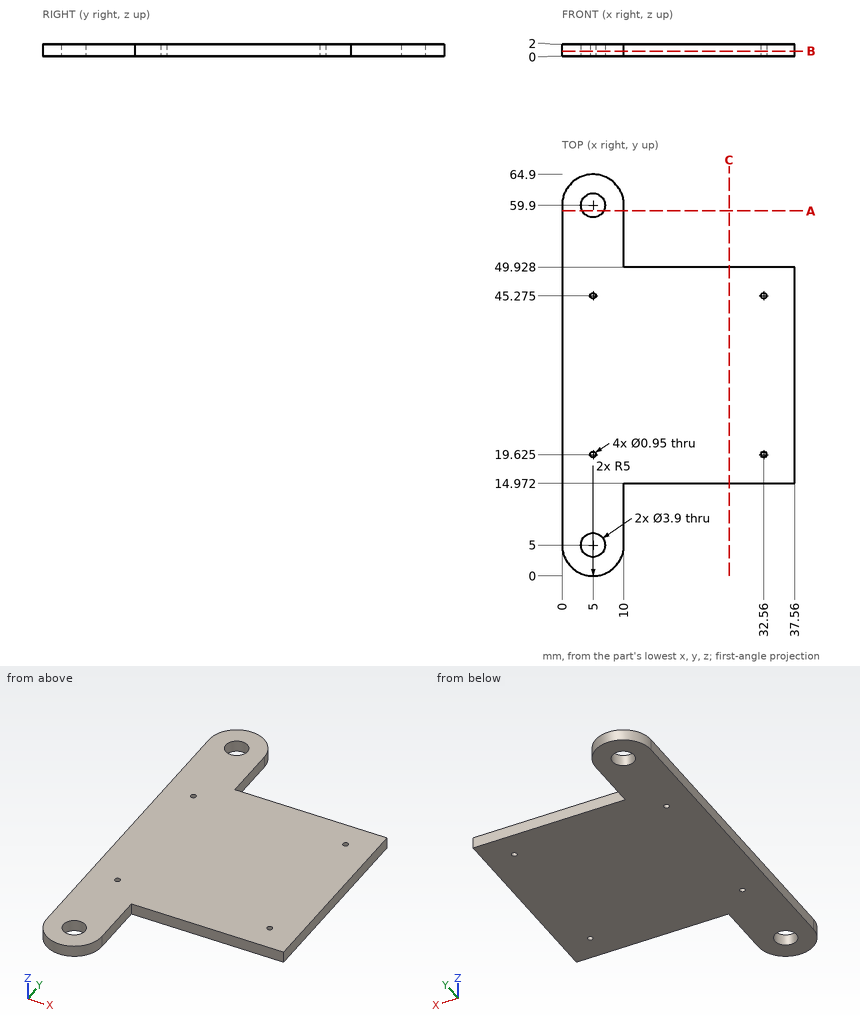
Can you work these out from the drawing? Everything is in mm from the part's minimum corner. Give positions to 0.01 mm unless a question says otherwise; leave off trailing zeros. Loops run counter-clockwise (first coordinate to the right, second up) from the corner with the lowest first, then second, coordinate; pieces in that order, holes last. Notation, with made-up numbers: (2, -40) - (12, -40) arc R18 cw to (12, -11) - close; hole circle Ø11 at (67, 65.25). An arc over 180 degrees is marked (long way). Answer as a JSON object with one key per item and string values.
Q1. Imagine slicing it at C-C on x = 27. Write out the boundary of the cut face in (y, z).
Geometry says:
{"outline": "(14.97, 0) - (49.93, 0) - (49.93, 2) - (14.97, 2) - close"}
Q2. If I drill on L1, parallel to Y at x = 5, z = 1.3; L2, parallel to Y at x = 32.56, z = 0.75; L3, parallel to Y at x = 6.5, z = 1.25 (1 decimal), over which ranges is the centre line in solid material (lowest first)?
Geometry says:
{"L1": "0 to 3.05, 6.95 to 19.15, 20.1 to 44.8, 45.75 to 57.95, 61.85 to 64.9", "L2": "14.97 to 19.15, 20.1 to 44.8, 45.75 to 49.93", "L3": "0.2 to 3.8, 6.2 to 58.7, 61.1 to 64.7"}
Q3. Imagine slicing it at B-B on z = 0.85. Give the number of separate pieces and of enclosed holes in the cut face, plus the area to 3 significant figures.
Geometry says:
{"separate pieces": "1", "enclosed holes": "6", "area": "1,560 mm²"}
Q4. Will these pins go through, and if not, where does the flat tip stop? P1, Ø10, axis at x = 21, y = 56.5, coming from the +Z side; P2, Ø1, axis at y = 9.5, z = 1, coming from the +X side; P3, Ø1, axis at x = 23.5, z = 2, coming from the +Y side; P4, Ø1, axis at x = 23, z = 1, coming from the -Y side.
Geometry says:
{"P1": "through", "P2": "x = 10", "P3": "y = 49.93", "P4": "y = 14.97"}
Q5. Imagine slicing it at A-A on y = 59. Write out the boundary of the cut face in (x, z).
Geometry says:
{"outline": "(0, 0) - (3.27, 0) - (3.27, 2) - (0, 2) - close; (6.73, 0) - (10, 0) - (10, 2) - (6.73, 2) - close"}
